Can you work these out from the drawing? Everything is in mm from the part's minimum corner. Round coordinates to 2 decimals unless told otherwise and drop trailing zeros. Loops run counter-clockwise (first coordinate to the right, second up) from the corner with the lowest first, then second, coordinate; pieces in that order, holes last. Notation, with made-up numbers: (3, 12) -> (20, 12) arc R13 ccw to (20, 29) -> close; hole circle Ø10 at (77, 61). An arc over 180 degrees is marked (long way). Answer as a JSON object with one key per item and string values.
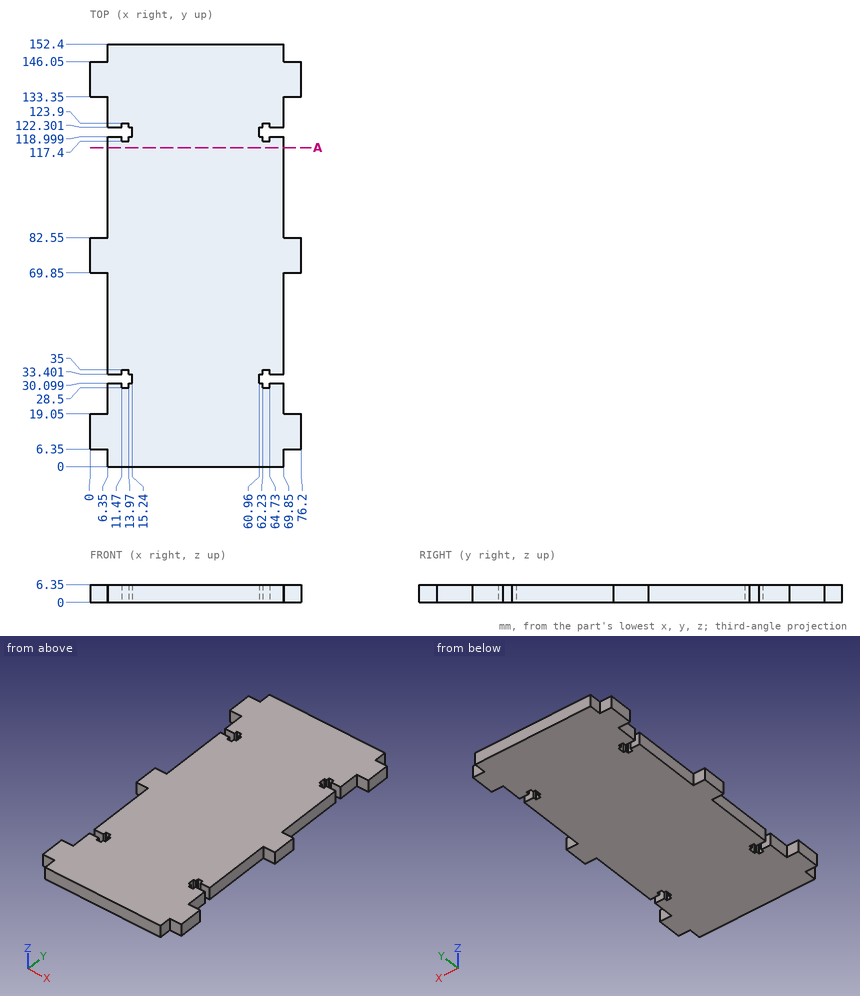
Q1. I'm going to push flat-ended pins straight in: pin 1 (2.5 mm diameter, centred on y = 31.5, z = 3.5, fed in from -X); pin 2 (1.3 mm diameter, centred on y = 123.5, z = 3.5, fed in from +X); pin 3 (1.9 mm diameter, centred on x = 2, z = 4, fed in from -Y). Where does each tip first touch, or does it pass through?
Determined:
{"pin 1": "x = 15.24", "pin 2": "x = 69.85", "pin 3": "y = 6.35"}
Q2. I want a section at A-A, the plane y = 115. Write out the boundary of the cut face in (x, z), then the cut area to 3 significant figures.
Determined:
{"outline": "(6.35, 0) -> (69.85, 0) -> (69.85, 6.35) -> (6.35, 6.35) -> close", "area": "403 mm²"}
Q3. If I drill on L1, parallel to Y at x = 15, z = 1.75; L2, parallel to X at y = 123.5, z = 0.5; L3, parallel to Y at x = 5.5, z = 1.5, over which ranges is the centre line in solid material (lowest first)? Write a range as [from, to].
Determined:
{"L1": "[0, 30.1], [33.4, 119], [122.3, 152.4]", "L2": "[6.35, 11.47], [13.97, 62.23], [64.73, 69.85]", "L3": "[6.35, 19.05], [69.85, 82.55], [133.35, 146.05]"}
